Could you check a few things on this model? Use its own coordinates, in mm. Coordinates: 2 decimals unless noted, no trailing zeros. Answer as CSV lines item,"result". Start each with the question number.
Item 1: If I drill on line 1 along X through (y, z) = (-9.5, 1.55); line 2 along Y through (x, z) = (4.5, 3.75); line 3 along Y through (x, z) = (7, 1.5), over which ranges is the centre line in solid material (lowest first)? Write a range as [from, to].
Item 2: I'm going to push flat-ended pins straight in: P1, Ø2, axis at y = -4, z = 2, coming from the +X side; P2, Ø1.5, axis at x = 5.5, z = 3.5, coming from the +Y side; P3, Ø1, axis at x = 4, z = 2.5, coming from the -Y side. Where does each tip first touch, or does it pass through?
Item 3: We'd pull the mould along X, two halves only. Please class faces 1 (the cylindrical face through (8.59, -9.49, 2.22)), 2 (the flat face through (3.5, -7, 4.5)): +X half, -X half, draft (parallel to the pull), parting line (faces both ways), or undercut.
```python
from build123d import *

# Parameters (mm, degrees)
F0_W     = 14
F0_H     = 14
F1_DEPTH = 4.5
F1_TAPER = -8
F2_R     = 1
F3_R     = 2.9535288369
F4_DEPTH = 25


with BuildPart() as f1:
    # F0 (on Top) → F1 (new body)
    with BuildSketch(Plane.XY):
        with Locations((7, -7)):
            Rectangle(F0_W, F0_H)
    extrude(amount=F1_DEPTH, taper=F1_TAPER)

    # F2
    f2_edges = [f1.edges().sort_by_distance(p)[0] for p in [
        (-0.316217, -14.316217, 2.25),
        (14.316217, -14.316217, 2.25),
        (14.316217, 0.316217, 2.25),
        (-0.316217, 0.316217, 2.25),
    ]]
    fillet(f2_edges, radius=F2_R)

    # F3 (on face) → F4 (cut)
    with BuildSketch(Plane(origin=(0, 0, 0), x_dir=(1, 0, 0), z_dir=(0, 0, -1))):
        with Locations((7, 7)):
            Circle(F3_R)
    extrude(amount=-F4_DEPTH, mode=Mode.SUBTRACT)


solid = f1.part
```
Ans:
1,line 1,"x = [-0.22, 5.43], [8.57, 14.22]"
1,line 2,"y = [-14.53, -8.57], [-5.43, 0.53]"
1,line 3,"y = [-14.21, -9.95], [-4.05, 0.21]"
2,P1,"stops at x = 14.42"
2,P2,"stops at y = 0.6"
2,P3,"stops at y = -14.42"
3,face 1,"undercut"
3,face 2,"draft"
